For this review, take the finished solid that the model builds, in its own axes (mm). Give positions to 0.01 mm unless a question says otherwise; leave off trailing zeros. Order: outer loops, then holes, each group sorted by start corner. A loop starts at its lowest first (then second) coordinate and runs counter-clockwise, first axis right, second up. Notation, with made-up numbers: (24.25, 88) - (34.25, 88) arc R21 cw to (34.25, 103) - close; hole circle Ø4 at (-18.5, -16). An arc over 180 degrees is marked (long way). Use a Markdown table: item, result. Add a question column.
1) We need section C-C on y = -899.5. Write out the cut boundary in (x, z), then the cut area to 3 significant figures.
2) Clearance check with flat-ended pins moving along their axes: P1, Ø8, axis at x = 12.5, y = -106, coming from the -Z side; P2, Ø1.5, axis at x = -12.5, z = -2.5, coming from the -Y side; P3, Ø1.5, axis at x = -1.5, z = 16, coming from the +Y side. State where each tip first meets the part, or that it passes through.
3) We need section A-A on z = 0. Write out the cut boundary in (x, y), then the cut area to 3 significant figures.
4) We need section B-B on x = 0. Write out the cut boundary in (y, z), then the cut area to 3 significant figures.
5) Wall thickness on L1, parallel to Y at x = 13, z = 1; L2, parallel to Y at x = 6, z = 8; L3, parallel to Z at x = 2.5, y = -450.5: over which ranges is each line inside the solid? List them lowest first.
```python
from build123d import *

# Parameters (mm, degrees)
F0_R     = 20
F1_DEPTH = 955
F2_R     = 11.254602
F3_DEPTH = 15
F4_R     = 11.5
F5_DEPTH = 15
F6_R     = 8.5
F7_DEPTH = 12
F8_R     = 8.5
F9_DEPTH = 12


with BuildPart() as f1:
    # F0 (on Front) → F1 (new body)
    with BuildSketch(Plane.XZ):
        Circle(F0_R)
    extrude(amount=F1_DEPTH)

    # F2 (on face) → F3 (join)
    with BuildSketch(Plane.XZ.offset(955)):
        Circle(F2_R)
    extrude(amount=F3_DEPTH)

    # F4 (on face) → F5 (join)
    with BuildSketch(Plane(origin=(0, 0, 0), x_dir=(-1, 0, 0), z_dir=(0, 1, 0))):
        Circle(F4_R)
    extrude(amount=F5_DEPTH)

    # F6 (on face) → F7 (join)
    with BuildSketch(Plane.XZ.offset(970)):
        Circle(F6_R)
    extrude(amount=F7_DEPTH)

    # F8 (on face) → F9 (join)
    with BuildSketch(Plane(origin=(0, 15, 0), x_dir=(-1, 0, 0), z_dir=(0, 1, 0))):
        Circle(F8_R)
    extrude(amount=F9_DEPTH)


solid = f1.part
```
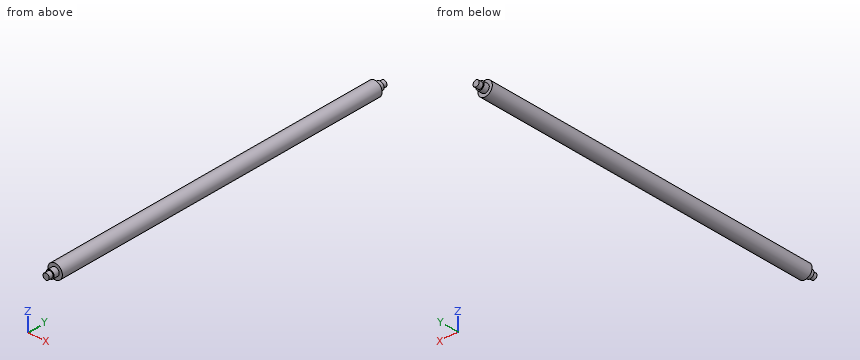
Checked values:
| question | item | result |
|---|---|---|
| 1 | outline | circle Ø40 at (0, 0) |
| 1 | area | 1,260 mm² |
| 2 | P1 | z = -18.1 |
| 2 | P2 | y = -955 |
| 2 | P3 | y = 0 |
| 3 | outline | (-20, -955) - (-11.25, -955) - (-11.25, -970) - (-8.5, -970) - (-8.5, -982) - (8.5, -982) - (8.5, -970) - (11.25, -970) - (11.25, -955) - (20, -955) - (20, 0) - (11.5, 0) - (11.5, 15) - (8.5, 15) - (8.5, 27) - (-8.5, 27) - (-8.5, 15) - (-11.5, 15) - (-11.5, 0) - (-20, 0) - close |
| 3 | area | 39,300 mm² |
| 4 | outline | (-982, -8.5) - (-970, -8.5) - (-970, -11.25) - (-955, -11.25) - (-955, -20) - (0, -20) - (0, -11.5) - (15, -11.5) - (15, -8.5) - (27, -8.5) - (27, 8.5) - (15, 8.5) - (15, 11.5) - (0, 11.5) - (0, 20) - (-955, 20) - (-955, 11.25) - (-970, 11.25) - (-970, 8.5) - (-982, 8.5) - close |
| 4 | area | 39,300 mm² |
| 5 | L1 | -955 to 0 |
| 5 | L2 | -970 to 15 |
| 5 | L3 | -19.84 to 19.84 |
